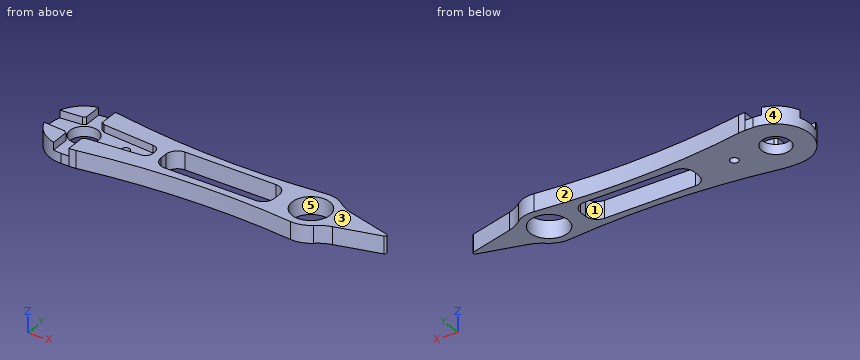
```python
from build123d import *

# Parameters (mm, degrees)
ESQUISSE1_R             = 3.75
ESQUISSE1_R_2           = 1.6
ESQUISSE1_R_3           = 1.1
BOSS_EXTRU_1_DEPTH      = 2.6
ESQUISSE2_R             = 3.75
ESQUISSE2_R_2           = 1.6
ESQUISSE2_R_3           = 1.1
BOSS_EXTRU_2_DEPTH      = 2
ENL_V_MAT_EXTRU_1_DEPTH = 2
ENL_V_MAT_EXTRU_2_DEPTH = 41.288459886
CONG_1_R                = 2
CONG_2_R                = 10
ESQUISSE6_W             = 30
ESQUISSE6_H             = 7.96998198
ENL_V_MAT_EXTRU_4_DEPTH = 10
CONG_3_R                = 3
BOSS_EXTRU_3_DEPTH      = 4.6
CONG_4_R                = 0.5
ESQUISSE9_R             = 5
ENL_V_MAT_EXTRU_7_DEPTH = 52.019355151
CONG_5_R                = 10


with BuildPart() as part:
    # Esquisse1 → Boss.-Extru.1 (new body)
    with BuildSketch(Plane.XY):
        with BuildLine():
            Line((-30, 9), (30, 9))
            ThreePointArc((30, 9), (39, 0), (30, -9))
            Line((30, -9), (-30, -9))
            ThreePointArc((-30, -9), (-39, 0), (-30, 9))
        make_face()
        with Locations((-30, 0)):
            Circle(ESQUISSE1_R, mode=Mode.SUBTRACT)
        with Locations((30, 0)):
            Circle(ESQUISSE1_R_2, mode=Mode.SUBTRACT)
        with Locations((-19, 0)):
            Circle(ESQUISSE1_R_3, mode=Mode.SUBTRACT)
    extrude(amount=BOSS_EXTRU_1_DEPTH)

    # Esquisse2 → Boss.-Extru.2 (add)
    with BuildSketch(Plane.XY.offset(2.6)):
        with BuildLine():
            Line((-30, -9), (30, -9))
            ThreePointArc((30, -9), (39, 0), (30, 9))
            Line((30, 9), (-30, 9))
            ThreePointArc((-30, 9), (-39, 0), (-30, -9))
        make_face()
        with Locations((-30, 0)):
            Circle(ESQUISSE2_R, mode=Mode.SUBTRACT)
        with Locations((30, 0)):
            Circle(ESQUISSE2_R_2, mode=Mode.SUBTRACT)
        with Locations((-19, 0)):
            Circle(ESQUISSE2_R_3, mode=Mode.SUBTRACT)
    extrude(amount=BOSS_EXTRU_2_DEPTH)

    # Esquisse3 → Enlèv. mat.-Extru.1 (cut)
    with BuildSketch(Plane.XY.offset(4.6)):
        with BuildLine():
            Line((-32.1, 3.979949748), (-32.1, 11))
            Line((-32.1, 11), (-27.9, 11))
            Line((-27.9, 11), (-27.9, 3.979949748))
            ThreePointArc((-27.9, 3.979949748), (-27.524129159, 3.757667305), (-27.171572875, 3.5))
            Line((-27.171572875, 3.5), (-11.5, 2.25))
            Line((-11.5, 2.25), (-11.5, -2.25))
            Line((-11.5, -2.25), (-27.171572875, -3.5))
            ThreePointArc((-27.171572875, -3.5), (-27.524129159, -3.757667305), (-27.9, -3.979949748))
            Line((-27.9, -3.979949748), (-27.9, -11))
            Line((-27.9, -11), (-32.1, -11))
            Line((-32.1, -11), (-32.1, -3.979949748))
            ThreePointArc((-32.1, -3.979949748), (-32.475870841, -3.757667305), (-32.828427125, -3.5))
            Line((-32.828427125, -3.5), (-48.5, -2.25))
            Line((-48.5, -2.25), (-48.5, 2.25))
            Line((-48.5, 2.25), (-32.828427125, 3.5))
            ThreePointArc((-32.828427125, 3.5), (-32.475870841, 3.757667305), (-32.1, 3.979949748))
        make_face()
    extrude(amount=-ENL_V_MAT_EXTRU_1_DEPTH, mode=Mode.SUBTRACT)

    # Esquisse4 → Enlèv. mat.-Extru.2 (cut, through all)
    with BuildSketch(Plane.XY.offset(4.6)):
        with BuildLine():
            Line((-27, 9), (-27, 15.262477906))
            Line((-27, 15.262477906), (45.494284805, 15.262477906))
            Line((45.494284805, 15.262477906), (45.494284805, -15.262477906))
            Line((45.494284805, -15.262477906), (-27, -15.262477906))
            Line((-27, -15.262477906), (-27, -9))
            ThreePointArc((-27, -9), (1.06358338, -6), (29.270665078, -6.961901362))
            ThreePointArc((29.270665078, -6.961901362), (37, 0), (29.270665078, 6.961901362))
            ThreePointArc((29.270665078, 6.961901362), (1.06358338, 6), (-27, 9))
        make_face()
    extrude(amount=-ENL_V_MAT_EXTRU_2_DEPTH, mode=Mode.SUBTRACT)

    # Congé1
    cong_1_edges = [part.edges().sort_by_distance(p)[0] for p in [
        (-11.5, 2.25, 3.6),
        (-11.5, -2.25, 3.6),
    ]]
    fillet(cong_1_edges, radius=CONG_1_R)

    # Congé2
    cong_2_edges = [part.edges().sort_by_distance(p)[0] for p in [
        (-27, 9, 2.3),
        (-27, -9, 2.3),
    ]]
    fillet(cong_2_edges, radius=CONG_2_R)

    # Esquisse6 → Enlèv. mat.-Extru.4 (cut)
    with BuildSketch(Plane.XY.offset(4.6)):
        with Locations((6, 0)):
            Rectangle(ESQUISSE6_W, ESQUISSE6_H)
    extrude(amount=-ENL_V_MAT_EXTRU_4_DEPTH, mode=Mode.SUBTRACT)

    # Congé3
    cong_3_edges = [part.edges().sort_by_distance(p)[0] for p in [
        (-9, -3.98499099, 2.3),
        (-9, 3.98499099, 2.3),
        (21, 3.98499099, 2.3),
        (21, -3.98499099, 2.3),
    ]]
    fillet(cong_3_edges, radius=CONG_3_R)

    # Esquisse8 → Boss.-Extru.3 (add)
    with BuildSketch(Plane.XY.offset(4.6)):
        Polygon((51.444700397, 0), (35.567285724, 4.243268748), (35.567285724, -4.243268748), align=None)
    extrude(amount=-BOSS_EXTRU_3_DEPTH)

    # Congé4
    cong_4_edges = [part.edges().sort_by_distance(p)[0] for p in [
        (51.444700397, 0, 2.3),
    ]]
    fillet(cong_4_edges, radius=CONG_4_R)

    # Esquisse9 → Enlèv. mat.-Extru.7 (cut, through all)
    with BuildSketch(Plane.XY.offset(4.6)):
        with Locations((30, 0)):
            Circle(ESQUISSE9_R)
    extrude(amount=-ENL_V_MAT_EXTRU_7_DEPTH, mode=Mode.SUBTRACT)

    # Congé5
    cong_5_edges = [part.edges().sort_by_distance(p)[0] for p in [
        (35.567285724, -4.243268748, 2.3),
        (35.567285724, 4.243268748, 2.3),
    ]]
    fillet(cong_5_edges, radius=CONG_5_R)


solid = part.part
```
Can you work these out from the model? Positions are in its coordinate system, mm. Face numbers are marked on the shaded views. A direction names the side the tool comes from. Coordinates: 2 decimals unless noted, no trailing zeros. Loops run counter-clockwise (first coordinate to the right, second up) from the corner with the lowest first, then second, coordinate; pieces in that order, holes last.
1) I need wall thicknesses on probe 1 along Y at (x, z) = (-30, 1.4); probe 2 along Y at (x, z) = (30, 2.1); probe 3 along Y at (x, z) = (37.5, 2.35). Which ranges of each line are inside material? Lowest first, please.
2) Thinking about a two-plate mould opening in X: for the marked faces 3, 4 and 5, which applies, pulls with the +X half, pulls with the -X half, needs draft (parallel to the pull), parting line crosses it, or undercut?
3) Imagine slicing it at D-D on x = -19. List the corners of the cut face in (y, z) for me, plus the area to 3 significant figures.
4) For pin 1 (8 mm diameter, centred on x = 30, y = 0, fed in from +Z); pin 2 (0.6 mm diameter, centred on y = 6.5, z = 4, fed in from +X); pin 3 (2 mm diameter, centred on x = -18, z = 2.5, fed in from -Y); pin 4 (1.4 mm diameter, centred on x = 5, z = 1.5, fed in from -Y), each with a flat end and sliding along its axis, tell me the tip position at first contact or that it passes through.
5) Which directions (+Z, -Z, +X, -X, +Y, -Y) give clear straight access to the entire face, cutting with the end or side of a thin tool? Please do the marked faces 1 and 2.
6) Imagine slicing it at A-A on x = 30. List the corners of the cut face in (y, z) for me, plus the area to 3 significant figures.
7) Imagine slicing it at B-B on z = 3.55. State how many separate pieces and enclosed holes the cut face has, plus the area to 3 significant figures.
Completed:
1. probe 1: y = -9 to -3.75, 3.75 to 9
1. probe 2: y = -7 to -5, 5 to 7
1. probe 3: y = -3.75 to 3.75
2. face 3: needs draft
2. face 4: pulls with the -X half
2. face 5: undercut
3. outline: (-7.74, 0) - (-1.1, 0) - (-1.1, 2.6) - (-2.85, 2.6) - (-2.85, 4.6) - (-7.74, 4.6) - close; (1.1, 0) - (7.74, 0) - (7.74, 4.6) - (2.85, 4.6) - (2.85, 2.6) - (1.1, 2.6) - close
3. area: 54.1 mm2
4. pin 1: passes through
4. pin 2: stops at x = 33.25
4. pin 3: stops at y = -7.74
4. pin 4: stops at y = -5.91
5. face 1: +Z, -Z
5. face 2: +Z, -Z, +Y
6. outline: (-7, 0) - (-5, 0) - (-5, 4.6) - (-7, 4.6) - close; (5, 0) - (7, 0) - (7, 4.6) - (5, 4.6) - close
6. area: 18.4 mm2
7. separate pieces: 3
7. enclosed holes: 2
7. area: 553 mm2
